from build123d import *

# Parameters (mm, degrees)
SKETCH2_W           = 184.15
SKETCH2_H           = 50.8
BOSS_EXTRUDE1_DEPTH = 1.5875
SKETCH3_R           = 1.61
SKETCH3_W           = 7.62
SKETCH3_H           = 10.15
CUT_EXTRUDE1_DEPTH  = 5.08


with BuildPart() as part:
    # Sketch2 → Boss-Extrude1 (new body, symmetric)
    with BuildSketch(Plane.XY):
        Rectangle(SKETCH2_W, SKETCH2_H)
    extrude(amount=BOSS_EXTRUDE1_DEPTH, both=True)

    # Sketch3 → Cut-Extrude1 (cut)
    with BuildSketch(Plane.XY.offset(1.5875)):
        with Locations((-50.605000009, 18.64)):
            Circle(SKETCH3_R)
        with Locations((-50.605000009, -18.64)):
            Circle(SKETCH3_R)
        with Locations((50.605000009, 18.64)):
            Circle(SKETCH3_R)
        with Locations((50.605000009, -18.64)):
            Circle(SKETCH3_R)
        with Locations((-36.970000018, 0)):
            Rectangle(SKETCH3_W, SKETCH3_H)
        with Locations((64.24, 0)):
            Rectangle(SKETCH3_W, SKETCH3_H)
    extrude(amount=-CUT_EXTRUDE1_DEPTH, mode=Mode.SUBTRACT)


solid = part.part
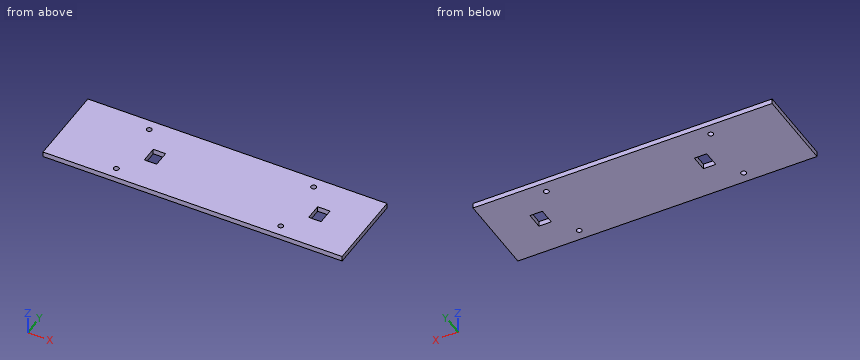
Design review of the part built by this model. Coordinates are the model's own, in mm. Round coordinates to 2 decimals unless told otherwise and drop trailing zeros. Order: outer loops, then holes, each group sorted by start corner. A loop starts at its lowest first (then second) coordinate and runs counter-clockwise, first axis right, second up. Notation, with made-up numbers: M -14.75,8 L 29.25,8 A23 ccw 29.25,46 Z; hole C 74,-38 d2. An arc over 180 degrees is marked long. Answer as CSV lines item,"result". Start each with the question number.
1) Add section C-C (y = 0.5). Give the number of separate pieces and of enclosed holes in the cut face, then the cut area to 3 significant figures.
2) Add section A-A (y = -18.64). Give the boundary of the cut face in (x, z) (1 decimal), then the cut area to 3 significant figures.
3) Add section B-B (z = -0.3). Give the boundary of the cut face in (x, y) (3 decimals), then the cut area to 3 significant figures.
4) Wall thickness on line 1 along X through (y, z) = (4, -1.1) (3 decimals); line 2 along X through (y, z) = (18.5, 1.2) (3 decimals); line 3 along Y through (x, z) = (63, 0.45) (3 decimals): over which ranges is each line inside the solid? List them lowest first. Write a range as [from, to].
Resolved:
1,separate pieces,"3"
1,enclosed holes,"0"
1,area,"536 mm^2"
2,outline,"M -92.1,-1.6 L -52.2,-1.6 L -52.2,1.6 L -92.1,1.6 Z; M -49,-1.6 L 49,-1.6 L 49,1.6 L -49,1.6 Z; M 52.2,-1.6 L 92.1,-1.6 L 92.1,1.6 L 52.2,1.6 Z"
2,area,"564 mm^2"
3,outline,"M -92.075,-25.4 L 92.075,-25.4 L 92.075,25.4 L -92.075,25.4 Z; hole C -50.605,-18.64 d3.22; hole C -50.605,18.64 d3.22; hole M -40.78,-5.075 L -33.16,-5.075 L -33.16,5.075 L -40.78,5.075 Z; hole C 50.605,-18.64 d3.22; hole C 50.605,18.64 d3.22; hole M 60.43,-5.075 L 68.05,-5.075 L 68.05,5.075 L 60.43,5.075 Z"
3,area,"9,170 mm^2"
4,line 1,"[-92.075, -40.78], [-33.16, 60.43], [68.05, 92.075]"
4,line 2,"[-92.075, -52.209], [-49.001, 49.001], [52.209, 92.075]"
4,line 3,"[-25.4, -5.075], [5.075, 25.4]"
